The drawing under review shows one solid part. Ordinate dimensions are in mm from its lowest x, y, z. A direction names the side the tool comes from. Round coordinates to 2 decimals unless told otherwise and drop trailing zeros. Write each loop counter-clockwise with the first axis right and the second up, starting at its lowest first coordinate (ties: lowest second). Pieces come first, ordered by that corner, then holes. Notation, with made-up numbers: (-17, 67) -> (-12, 67) arc R20 cw to (-12, 101) -> close; hole circle Ø4 at (38, 16). An arc over 180 degrees is marked (long way). Answer in a Markdown table with one row per item.
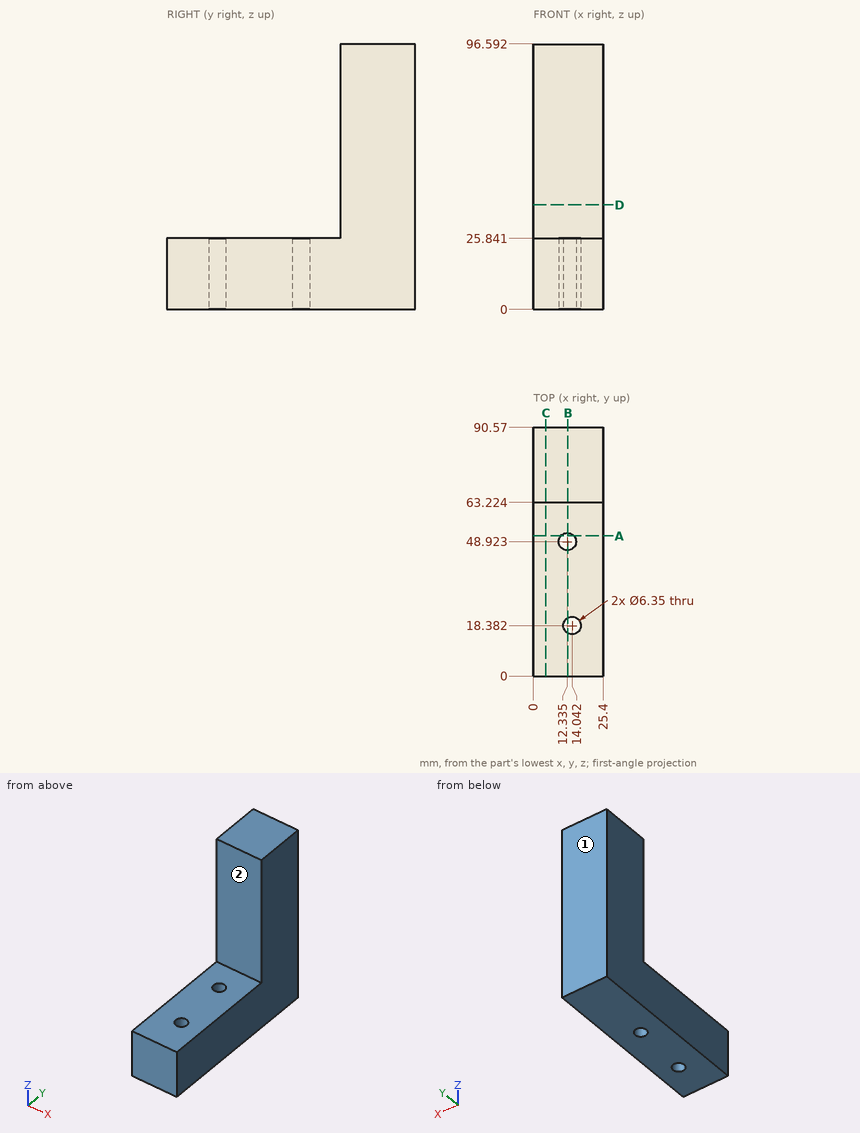
1) Clearance check with flat-ended pins moving along their axes: pin 1 Ø1 at (x, z) = (17.5, 29.5) entering from -Y; pin 2 Ø7.5 at (x, y) = (12.33, 48.92) entering from +Z. State where each tip first meets the part, or that it passes through.
Solved:
| item | result |
|---|---|
| pin 1 | y = 63.22 |
| pin 2 | z = 25.84 |
2) Consider section C-C on x = 4.5. State the section outline as (y, z) points.
Solved:
| item | result |
|---|---|
| outline | (0, 0) -> (90.57, 0) -> (90.57, 96.59) -> (63.22, 96.59) -> (63.22, 25.84) -> (0, 25.84) -> close |
3) For line 1 (Y direction, x = 2, z = 75.5); line 2 (Z direction, x = 3, y = 48), list the stretches that pass through material, from the lowest coordinate up. Write a range as [from, to].
Solved:
| item | result |
|---|---|
| line 1 | [63.22, 90.57] |
| line 2 | [0, 25.84] |
4) For the marked faces 1 and 2, list the 3-axis set-ups (+Z, -Z, +X, -X, +Y, -Y) from which the entire face can be reached by the end or side of a thin tool; tool diameter is ignored.
Solved:
| item | result |
|---|---|
| face 1 | +Z, -Z, +X, -X, +Y |
| face 2 | +Z, +X, -X, -Y |
5) Consider section D-D on z = 38. State the section outline as (x, y) points, then the cut area to 3 significant figures.
Solved:
| item | result |
|---|---|
| outline | (0, 63.22) -> (25.4, 63.22) -> (25.4, 90.57) -> (0, 90.57) -> close |
| area | 695 mm² |
6) Consider section A-A on y = 51. State the section outline as (x, z) points, then the cut area to 3 significant figures.
Solved:
| item | result |
|---|---|
| outline | (0, 0) -> (9.93, 0) -> (9.93, 25.84) -> (0, 25.84) -> close; (14.74, 0) -> (25.4, 0) -> (25.4, 25.84) -> (14.74, 25.84) -> close |
| area | 532 mm² |
7) Consider section B-B on x = 12.5. State the section outline as (y, z) points.
Solved:
| item | result |
|---|---|
| outline | (0, 0) -> (15.61, 0) -> (15.61, 25.84) -> (0, 25.84) -> close; (21.16, 0) -> (45.75, 0) -> (45.75, 25.84) -> (21.16, 25.84) -> close; (52.09, 0) -> (90.57, 0) -> (90.57, 96.59) -> (63.22, 96.59) -> (63.22, 25.84) -> (52.09, 25.84) -> close |
